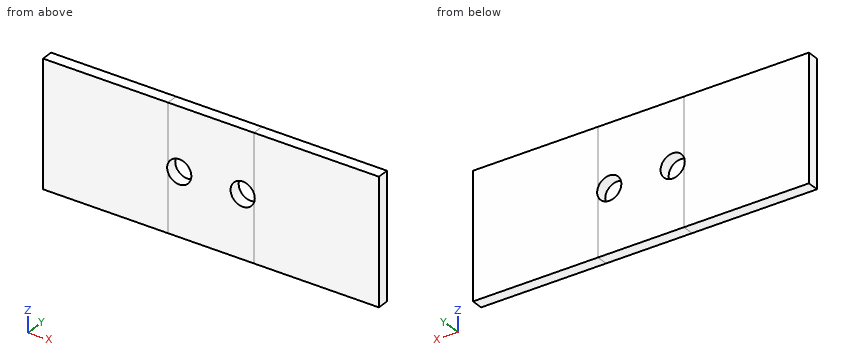
Autodesk Inventor part; units mm, degrees
ref_plane "Work Plane1" through (42.8625, 0, 0) normal (0, -1, 0) x (1, 0, 0)
ref_plane "YZ Plane" through (0, 0, 0) normal (1, 0, 0) x (0, 1, 0)
ref_plane "XZ Plane" through (0, 0, 0) normal (0, 1, 0) x (-1, 0, 0)
sketch "Sketch1" plane through (0, 0, 0) normal (0, 0, 1) x (1, 0, 0)
  line L0 (0, 0) -> (4.7625, 0)
  line L1 (4.7625, 3.1115) -> (3.9687, 3.1115) construction
  line L2 (0, 3.1115) -> (0, 0)
  line L3 (4.7625, 0) -> (12.7, 0)
  line L4 (12.7, 0) -> (12.7, 3.1115) construction
  line L5 (12.7, 5.1753) -> (11.1125, 5.1753) construction
  line L6 (4.7625, 5.1753) -> (4.7625, 3.1115) construction
  line L7 (2.3812, 3.1115) -> (2.3812, 0) construction
  line L8 (8.7312, 5.1753) -> (8.7312, 0) construction
  line L9 (2.3812, 3.1115) -> (2.3812, 5.4927) construction
  circle A0 centre (2.3812, 5.4927) radius 2.3812 construction
  line L10 (6.35, 5.1753) -> (6.35, 0) construction
  line L11 (11.1125, 5.1753) -> (11.1125, 0) construction
  line L12 (4.7625, 3.1115) -> (12.7, 3.1115) construction
  line L13 (6.35, 5.1753) -> (4.7625, 5.1753) construction
  line L14 (4.7625, 3.1115) -> (4.7625, 0) construction
  line L15 (11.1125, 5.1753) -> (10.3187, 5.1753) construction
  line L16 (12.7, 3.1115) -> (12.7, 5.1753) construction
  line L17 (8.7312, 5.1753) -> (8.7312, 7.5565) construction
  circle A1 centre (8.7312, 7.5565) radius 2.3813 construction
  line L18 (0.7937, 3.1115) -> (0.7937, 0)
  line L19 (3.9687, 3.1115) -> (3.9687, 0)
  line L20 (7.1437, 5.1753) -> (7.1437, 0)
  line L21 (10.3187, 5.1753) -> (10.3187, 0)
  line L22 (3.9687, 3.1115) -> (0.7937, 3.1115)
  line L23 (0.7937, 3.1115) -> (0, 3.1115)
  line L24 (10.3187, 5.1753) -> (8.7312, 5.1753)
  line L25 (7.1437, 5.1753) -> (6.35, 5.1753) construction
  line L26 (8.7312, 5.1753) -> (7.1437, 5.1753)
  line L27 (3.9687, 3.1115) -> (7.1437, 5.1753)
  line L28 (0, 0) -> (0, 5.5563) construction
  line L29 (0, 5.5563) -> (17.4625, 5.5563)
  line L30 (0, 5.5563) -> (0, 7.9375)
  line L31 (0, 7.9375) -> (17.4625, 7.9375)
  line L32 (12.7, 3.1115) -> (13.4937, 3.1115) construction
  line L33 (12.7, 0) -> (17.4625, 0)
  line L34 (17.4625, 0) -> (17.4625, 3.1115)
  line L35 (15.0812, 0) -> (15.0812, 3.1115) construction
  line L36 (13.4937, 3.1115) -> (13.4937, 0)
  line L37 (16.6687, 3.1115) -> (16.6687, 0)
  line L38 (13.4937, 3.1115) -> (15.0812, 3.1115)
  line L39 (16.6687, 3.1115) -> (17.4625, 3.1115)
  line L40 (15.0812, 3.1115) -> (16.6687, 3.1115)
  line L41 (15.0812, 3.1115) -> (15.0812, 5.4928) construction
  circle A2 centre (15.0812, 5.4928) radius 2.3813 construction
  line L42 (10.3187, 5.1753) -> (13.4937, 3.1115)
  line L43 (0, -12.7) -> (0, 0) construction
  line L44 (0, -7.1437) -> (26.1938, -7.1437) construction
  line L45 (0, -4.7625) -> (26.1938, -4.7625) construction
  line L46 (26.1938, -4.7625) -> (26.1938, -7.1437) construction
  line L47 (26.1938, -7.1437) -> (26.1938, -12.7) construction
  line L48 (26.1938, -12.7) -> (0, -12.7) construction
  line L49 (26.1938, -6.35) -> (34.3852, -6.35) construction
  line L50 (26.1938, -12.7) -> (34.3852, -12.7) construction
  line L51 (34.3852, -12.7) -> (34.3852, -6.35) construction
  line L52 (16.6688, -4.7625) -> (16.6688, -12.7) construction
  circle A3 centre (16.6688, -5.1435) radius 2.3813 construction
  circle A4 centre (16.6688, -7.2073) radius 2.3813 construction
  circle A5 centre (10.3187, -5.1435) radius 2.3813 construction
  circle A6 centre (10.3187, -7.2073) radius 2.3813 construction
  line L53 (10.3187, -4.7625) -> (10.3187, -12.7) construction
  line L54 (0, -7.5248) -> (26.1938, -7.5248) construction
  line L55 (8.7312, -7.5248) -> (8.7312, -12.7) construction
  line L56 (5.5562, -7.5248) -> (5.5562, -12.7) construction
  line L57 (18.2563, -7.5248) -> (18.2563, -12.7) construction
  line L58 (21.4313, -7.5248) -> (21.4313, -12.7) construction
  line L59 (0, -9.5885) -> (26.1938, -9.5885) construction
  line L60 (5.5562, -9.5885) -> (8.7312, -7.5248) construction
  line L61 (18.2563, -7.5248) -> (21.4312, -9.5885) construction
  line L62 (11.9062, -7.5248) -> (11.9062, -12.7) construction
  line L63 (15.0812, -7.5248) -> (15.0812, -12.7) construction
  line L64 (11.9062, -7.5248) -> (15.0812, -9.5885) construction
  line L65 (21.4313, -9.3266) -> (34.3852, -9.3266) construction
  line L66 (24.6063, -9.3266) -> (24.6063, -12.7) construction
  line L67 (21.4313, -9.3266) -> (20.1197, -7.1437) construction
  line L68 (26.1938, -9.5885) -> (30.9563, -9.5885) construction
  line L69 (30.9563, -9.5885) -> (30.9563, -12.7) construction
  line L70 (31.75, -9.3266) -> (31.75, -12.7) construction
  line L71 (31.75, -12.7) -> (29.723, -9.3266) construction
  line L72 (0, -4.7625) -> (-1.5875, -4.7625) construction
  line L73 (-1.5875, -4.7625) -> (-1.5875, -9.3266) construction
  line L74 (-1.5875, -9.3266) -> (5.5562, -9.3266) construction
  line L75 (1.4233, 7.874) -> (3.7622, 7.874)
  line L76 (17.4625, 5.5563) -> (17.4625, 7.9375)
  dimension "d8" = 6.35
  dimension "d9" = 5.1753
  dimension "d10" = 4.7625
  dimension "d11" = 2.3813
  dimension "d12" = 3.175
  dimension "d13" = 3.175
  dimension "d14" = 4.7625
  dimension "d15" = 2.3813
  dimension "d16" = 3.1115
  dimension "d17" = 5.5563
  dimension "d18" = 7.9375
  dimension "d19" = 6.35
  dimension "d20" = 3.175
  dimension "d21" = 2.3813
  dimension "d25" = 12.7
  dimension "d26" = 5.5563
  dimension "d27" = 7.9375
  dimension "d28" = 26.1938
  dimension "d29" = 8.1915
  dimension "d30" = 6.35
  dimension "d33" = 9.525
  dimension "d35" = 0.381
  dimension "d36" = 0.0635
  dimension "d38" = 6.35
  dimension "d39" = 0.381
  dimension "d40" = 0.381
  dimension "d41" = 0.0635
  dimension "d42" = 0.0635
  dimension "d43" = 9.525
  dimension "d46" = 1.5875
  dimension "d47" = 4.7625
  dimension "d48" = 1.5875
  dimension "d49" = 4.7625
  dimension "d50" = 3.1115
  dimension "d51" = 1.5875
  dimension "d52" = 4.7625
  dimension "d53" = 3.3734
  dimension "d54" = 3.175
  dimension "d55" = 31
  dimension "d56" = 9.525
  dimension "d57" = 9.525
  dimension "d59" = 0.7937
  dimension "d60" = 31
  dimension "d61" = 1.5875
  dimension "d62" = 3.3734
  dimension "d63" = 0.0635
extrude "Extrusion1" add sketch "Sketch1" along normal blind 25.4 contours L30 L31 L76 L29
sketch "Sketch2" plane through (17.4625, 5.5563, 0) normal (1, 0, 0) x (0, 0, -1)
  line L0 (0, 0) -> (0, 2.3813)
  line L1 (0, 2.3813) -> (-25.4, 2.3813)
  line L2 (-25.4, 0) -> (-25.4, 2.3813)
  line L3 (0, 0) -> (-25.4, 0)
  point P0 (0, -5.5562)
extrude "Extrusion3" add sketch "Sketch2" along normal blind 25.4
sketch "Sketch4" plane through (0, 5.5563, 0) normal (-1, 0, 0) x (0, 0, 1)
  line L0 (0, 2.3812) -> (0, 0)
  line L1 (0, 0) -> (25.4, 0)
  line L2 (25.4, 2.3812) -> (25.4, 0)
  line L3 (0, 2.3812) -> (25.4, 2.3812)
  point P0 (0, -5.5563)
extrude "Extrusion4" add sketch "Sketch4" along normal blind 25.4
sketch "Sketch3" plane through (0, 7.9375, 0) normal (0, 1, 0) x (1, 0, 0)
  line L0 (0, 0) -> (0, -25.4)
  line L1 (17.4625, 0) -> (17.4625, -25.4)
  circle A0 centre (2.286, -12.7) radius 2.4574
  circle A1 centre (15.1765, -12.7) radius 2.4574
  line L2 (0, -12.7) -> (17.4625, -12.7) construction
  dimension "d66" = 4.9149
  dimension "d67" = 12.8905
  dimension "d68" = 2.286
  dimension "d69" = 2.286
extrude "Extrusion2" cut sketch "Sketch3" against normal blind 25.4
ref_plane "Work Plane1" through (42.8625, 0, 0) normal (0, -1, 0) x (1, 0, 0)
equation "\"d19\" = d8"
equation "\"d26\" = d17"
equation "\"d27\" = d18"
equation "\"d39\" = d35"
equation "\"d40\" = d39"
equation "\"d41\" = d36"
equation "\"d42\" = d41"
equation "\"d50\" = d16"
equation "\"d51\" = d46"
equation "\"d52\" = d47"
equation "\"d57\" = d56"
equation "\"d60\" = d55"
equation "\"d62\" = d53"
equation "\"d68\" = d69"
properties part number "Sketch - Ball Shifting Shaft"
Could you check a few things on this model? Use its own coordinates, in mm. Give positions to 0.01 mm unless a question says otherwise; leave off trailing zeros. Order: outer loops, then holes, each group sorted by start corner. A loop starts at its lowest first (then second) coordinate and runs counter-clockwise, first axis right, second up. Notation, with made-up numbers: (31.5, -35) - (55.5, -35) arc R23 ccw to (55.5, -10) - close; hole circle Ø10 at (33.25, -30). An arc over 180 degrees is marked (long way). Return JSON: item names as keys, results as strings. Group by question number.
Q1. Suppose I cut it at A-A, the plane z = 12.7. Please give me the cut outline in (x, y), and give its area (3 significant figures).
Q2. Suppose I cut it at C-C, the plane x = 14.5. Please give me the cut outline in (y, z).
Q3. Please list where these lines run through material, in increasing order: line 1 along X through (y, z) = (6.4, 12.7); line 2 along X through (y, z) = (7.3, 10.5). Write a range as [from, to].
Q4. Suppose I cut it at B-B, the plane y = 7.4. Please give me the cut outline in (x, z), and give its area (3 significant figures).
Resolved:
{
 "1": {"outline": "(-25.4, 5.56) - (-0.17, 5.56) - (-0.17, 7.94) - (-25.4, 7.94) - close; (4.74, 5.56) - (12.72, 5.56) - (12.72, 7.94) - (4.74, 7.94) - close; (17.63, 5.56) - (42.86, 5.56) - (42.86, 7.94) - (17.63, 7.94) - close", "area": "139 mm2"},
 "2": {"outline": "(5.56, 0) - (7.94, 0) - (7.94, 10.34) - (5.56, 10.34) - close; (5.56, 15.06) - (7.94, 15.06) - (7.94, 25.4) - (5.56, 25.4) - close"},
 "3": {"line 1": "x = [-25.4, -0.17], [4.74, 12.72], [17.63, 42.86]", "line 2": "x = [-25.4, 1.19], [3.38, 14.08], [16.27, 42.86]"},
 "4": {"outline": "(-25.4, 0) - (42.86, 0) - (42.86, 25.4) - (-25.4, 25.4) - close; hole circle Ø4.91 at (2.29, 12.7); hole circle Ø4.91 at (15.18, 12.7)", "area": "1,700 mm2"}
}
